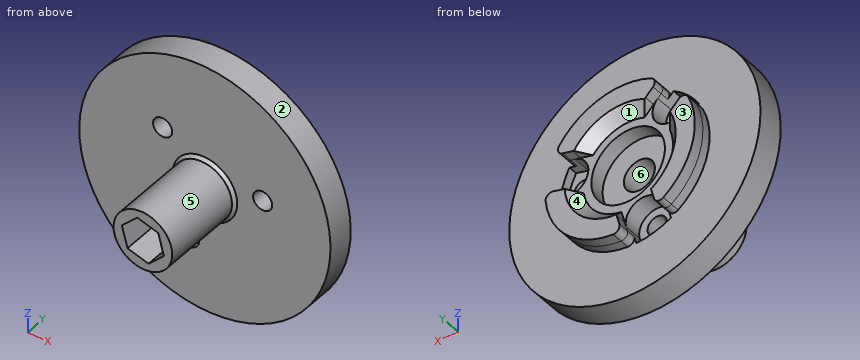
```python
from build123d import *
from build123d.topology import SkipClean

# Parameters (mm, degrees)
SKETCH_1_R               = 4
SKETCH_1_R_2             = 2.625
EXTRUDE_1_DEPTH          = 6
SKETCH_2_R               = 12.5
SKETCH_2_R_2             = 2.6
EXTRUDE_2_DEPTH          = 6
SKETCH_3_R               = 1.6
CUT_EXTRUDE_1_DEPTH      = 15
SKETCH_6_R               = 1.6
CUT_EXTRUDE_5_DEPTH      = 3
PATTERN_CIRCULAR_1_COUNT = 3
EXTRUDE_START            = 13.8
SKETCH_4_R               = 4.9
SKETCH_4_R_2             = 2.6
EXTRUDE_3_DEPTH          = 13.8
SKETCH_7_R               = 6.15
CUT_EXTRUDE_7_DEPTH      = 2.5
CUT_EXTRUDE_8_DEPTH      = 12.55
SKETCH_10_R              = 21
SKETCH_10_R_2            = 12.5
EXTRUDE_4_DEPTH          = 4.5
EXTRUDE_5_DEPTH          = 1.8
PATTERN_CIRCULAR_2_COUNT = 3
FILLET_1_R               = 1
CHAMFER_1_SIZE           = 0.5
CHAMFER_2_SIZE           = 2


with BuildPart() as part:
    # 草图1 → 凸台-拉伸1 (new body)
    with BuildSketch(Plane(origin=(0, 0, 0), x_dir=(1, 0, 0), z_dir=(0, 1, 0))):
        with Locations(Location((0, 0, 0), (0, 0, 270))):
            Circle(SKETCH_1_R)
        with Locations(Location((0, 0, 0), (0, 0, 270))):
            Circle(SKETCH_1_R_2, mode=Mode.SUBTRACT)
    extrude(amount=EXTRUDE_1_DEPTH)

    # 草图2 → 凸台-拉伸2 (add)
    with BuildSketch(Plane(origin=(0, 0, 0), x_dir=(-1, 0, 0), z_dir=(0, -1, 0))):
        with Locations(Location((0, 0, 0), (0, 0, 90))):
            Circle(SKETCH_2_R)
        with Locations(Location((0, 0, 0), (0, 0, 90))):
            Circle(SKETCH_2_R_2, mode=Mode.SUBTRACT)
    extrude(amount=-EXTRUDE_2_DEPTH)

    # 草图3 → 切除-拉伸1 (cut)
    with BuildSketch(Plane(origin=(0, 6, 0), x_dir=(1, 0, 0), z_dir=(0, 1, 0))):
        with Locations(Location((-2.588190451, 9.659258263, 0), (0, 0, 270))):
            Circle(SKETCH_3_R)
    cut_extrude_1 = extrude(amount=-CUT_EXTRUDE_1_DEPTH, mode=Mode.SUBTRACT)

    # 草图6 → 切除-拉伸5 (cut)
    with BuildSketch(Plane(origin=(0, 6, 0), x_dir=(1, 0, 0), z_dir=(0, 1, 0))):
        with BuildLine():
            Line((-6.038458877, 10.944725414), (-5.48596793, 8.882801128))
            ThreePointArc((-5.48596793, 8.882801128), (-1.811733316, 6.761480784), (0.309587028, 10.435715398))
            Line((0.309587028, 10.435715398), (-0.24290392, 12.497639685))
            ThreePointArc((-0.24290392, 12.497639685), (-3.235238064, 12.074072829), (-6.038458877, 10.944725414))
        make_face()
        with Locations(Location((-2.588190451, 9.659258263, 0), (0, 0, 270))):
            Circle(SKETCH_6_R, mode=Mode.SUBTRACT)
    cut_extrude_5 = extrude(amount=-CUT_EXTRUDE_5_DEPTH, mode=Mode.SUBTRACT)

    # 阵列(圆周)1: 切除-拉伸1, 切除-拉伸5 ×3 about axis
    pattern_circular_1_axis = Axis((0, 0, 0), (0, 1, 0))
    add([cut_extrude_1.rotate(pattern_circular_1_axis, i * 360 / PATTERN_CIRCULAR_1_COUNT) for i in range(1, PATTERN_CIRCULAR_1_COUNT)], mode=Mode.SUBTRACT)
    add([cut_extrude_5.rotate(pattern_circular_1_axis, i * 360 / PATTERN_CIRCULAR_1_COUNT) for i in range(1, PATTERN_CIRCULAR_1_COUNT)], mode=Mode.SUBTRACT)

    # 草图4 → 凸台-拉伸3 (add)
    with BuildSketch(Plane(origin=(0, 0, 0), x_dir=(-1, 0, 0), z_dir=(0, -1, 0)).offset(EXTRUDE_START)):
        with Locations(Location((0, 0, 0), (0, 0, 270))):
            Circle(SKETCH_4_R)
        with Locations(Location((0, 0, 0), (0, 0, 90))):
            Circle(SKETCH_4_R_2, mode=Mode.SUBTRACT)
    extrude(amount=-EXTRUDE_3_DEPTH)

    # 草图7 → 切除-拉伸7 (cut)
    with BuildSketch(Plane(origin=(0, 6, 0), x_dir=(1, 0, 0), z_dir=(0, 1, 0))):
        with Locations(Location((0, 0, 0), (0, 0, 270))):
            Circle(SKETCH_7_R)
    extrude(amount=-CUT_EXTRUDE_7_DEPTH, mode=Mode.SUBTRACT)

    # 草图8 → 切除-拉伸8 (cut)
    with BuildSketch(Plane(origin=(0, -13.8, 0), x_dir=(-1, 0, 0), z_dir=(0, -1, 0))):
        Polygon((-2.57196423, -2.57196423), (0.941404246, -3.513368476), (3.513368476, -0.941404246), (2.57196423, 2.57196423), (-0.941404246, 3.513368476), (-3.513368476, 0.941404246), align=None)
    extrude(amount=-CUT_EXTRUDE_8_DEPTH, mode=Mode.SUBTRACT)

    # 草图10 → 凸台-拉伸4 (add)
    with BuildSketch(Plane(origin=(0, 0, 0), x_dir=(1, 0, 0), z_dir=(0, 1, 0))):
        with Locations(Location((0, 0, 0), (0, 0, 270))):
            Circle(SKETCH_10_R)
        Circle(SKETCH_10_R_2, mode=Mode.SUBTRACT)
    extrude(amount=EXTRUDE_4_DEPTH)

    # 草图11 → 凸台-拉伸5 (add)
    with BuildSketch(Plane(origin=(0, 6, 0), x_dir=(1, 0, 0), z_dir=(0, 1, 0))):
        with BuildLine():
            Line((-5.230740824, 7.930280602), (-6.038458877, 10.944725414))
            ThreePointArc((-6.038458877, 10.944725414), (-12.074072829, 3.235238064), (-10.701821494, -6.459180807))
            Line((-10.701821494, -6.459180807), (-8.495094736, -4.252454048))
            ThreePointArc((-8.495094736, -4.252454048), (-9.17629535, 2.458780928), (-5.230740824, 7.930280602))
        make_face()
    extrude_5 = extrude(amount=EXTRUDE_5_DEPTH)

    # 阵列(圆周)2: 凸台-拉伸5 ×3 about axis
    with SkipClean():  # the faces are left unmerged after this step: merging them gives an invalid solid
        pattern_circular_2_axis = Axis((0, 3.5, 0), (0, 1, 0))
        for i in range(1, PATTERN_CIRCULAR_2_COUNT):
            add(extrude_5.rotate(pattern_circular_2_axis, i * 360 / PATTERN_CIRCULAR_2_COUNT))

    # 圆角1
    fillet_1_edges = [part.edges().sort_by_distance(p)[0] for p in [
        (-10.701821494, 6.9, 6.459180807),
        (-6.459180807, 6.9, 10.701821494),
        (10.944725414, 6.9, 6.038458877),
        (12.497639685, 6.9, 0.24290392),
        (-0.24290392, 6.9, -12.497639685),
        (-6.038458877, 6.9, -10.944725414),
    ]]
    fillet(fillet_1_edges, radius=FILLET_1_R)

    # 倒角1
    chamfer_1_edges = [part.edges().sort_by_distance(p)[0] for p in [
        (0, 0, -4.9),
    ]]
    chamfer(chamfer_1_edges, length=CHAMFER_1_SIZE)

    # 倒角2
    # the kernel refuses this chamfer: 2 mm, written as the material it adds along each edge
    with BuildSketch(Plane(origin=(0, 6, 0), x_dir=(-0.46364396793112084, 0, -0.8860215973671781), z_dir=(-0.8860215973671781, 0, 0.46364396793112084))) as chamfer_2_piece_1_section:
        Polygon((9.5 - CHAMFER_2_SIZE, 0), (9.5, -CHAMFER_2_SIZE), (9.5, 0), align=None)
    chamfer_2_piece_1 = revolve(axis=Axis((0, 6, 0), (0, -1, 0)), revolution_arc=145.244994466, mode=Mode.PRIVATE)
    chamfer_2_piece_1 = split(chamfer_2_piece_1, bisect_by=Plane(origin=(4.843261848, 6.879467901, -1.80808044), z_dir=(0.2588190451025276, 0, -0.9659258262890666)), keep=Keep.TOP, mode=Mode.PRIVATE)
    chamfer_2_piece_1 = split(chamfer_2_piece_1, bisect_by=Plane(origin=(1.80808044, 6.879467901, -4.843261848), z_dir=(0.9659258262890712, 0, -0.2588190451025102)), keep=Keep.TOP, mode=Mode.PRIVATE)
    chamfer_2_piece_1 = split(chamfer_2_piece_1, bisect_by=Plane(origin=(5.954215348, 7.8, -5.954215348), z_dir=(0, -1, 0)), keep=Keep.TOP, mode=Mode.PRIVATE)
    add(chamfer_2_piece_1)
    with BuildSketch(Plane(origin=(0, 6, 0), x_dir=(0.9991391955872041, 0, 0.04148334414382066), z_dir=(0.04148334414382066, 0, -0.9991391955872041))) as chamfer_2_piece_2_section:
        Polygon((9.5 - CHAMFER_2_SIZE, 0), (9.5, -CHAMFER_2_SIZE), (9.5, 0), align=None)
    chamfer_2_piece_2 = revolve(axis=Axis((0, 6, 0), (0, -1, 0)), revolution_arc=145.244994466, mode=Mode.PRIVATE)
    chamfer_2_piece_2 = split(chamfer_2_piece_2, bisect_by=Plane(origin=(3.290347577, 6.879467901, 3.987474517), z_dir=(-0.25881904510253106, 0, 0.9659258262890655)), keep=Keep.TOP, mode=Mode.PRIVATE)
    chamfer_2_piece_2 = split(chamfer_2_piece_2, bisect_by=Plane(origin=(-0.855787331, 6.879467901, 5.098428018), z_dir=(0.7071067811865428, 0, 0.7071067811865523)), keep=Keep.TOP, mode=Mode.PRIVATE)
    chamfer_2_piece_2 = split(chamfer_2_piece_2, bisect_by=Plane(origin=(2.179394077, 7.8, 8.133609425), z_dir=(0, -1, 0)), keep=Keep.TOP, mode=Mode.PRIVATE)
    add(chamfer_2_piece_2)
    with BuildSketch(Plane(origin=(0, 6, 0), x_dir=(-0.535495227656083, 0, 0.8445382532233574), z_dir=(0.8445382532233574, 0, 0.535495227656083))) as chamfer_2_piece_3_section:
        Polygon((9.5, -CHAMFER_2_SIZE), (9.5 - CHAMFER_2_SIZE, 0), (9.5, 0), align=None)
    chamfer_2_piece_3 = revolve(axis=Axis((0, 6, 0), (0, -1, 0)), revolution_arc=145.244994466, mode=Mode.PRIVATE)
    chamfer_2_piece_3 = split(chamfer_2_piece_3, bisect_by=Plane(origin=(-3.987474517, 6.879467901, -3.290347577), z_dir=(-0.96592582628907, 0, 0.25881904510251447)), keep=Keep.TOP, mode=Mode.PRIVATE)
    chamfer_2_piece_3 = split(chamfer_2_piece_3, bisect_by=Plane(origin=(-5.098428018, 6.879467901, 0.855787331), z_dir=(-0.7071067811865401, 0, -0.7071067811865549)), keep=Keep.TOP, mode=Mode.PRIVATE)
    chamfer_2_piece_3 = split(chamfer_2_piece_3, bisect_by=Plane(origin=(-8.133609425, 7.8, -2.179394077), z_dir=(0, -1, 0)), keep=Keep.TOP, mode=Mode.PRIVATE)
    add(chamfer_2_piece_3)


solid = part.part
```
CAD build for the part. Positions are in the model's coordinates, mm. Face numbers are marked on the shaded views. A direction names the side the tool comes from. Coordinates: 2 decimals unless noted, no trailing zeros. Order: outer loops, then holes, each group sorted by start corner. A loop starts at its lowest first (then second) coordinate and runs counter-clockwise, first axis right, second up. Notation, with made-up numbers: M -24.5,10.25 L 16.5,10.25 A24 cw 16.5,32.25 Z; hole C 35,-16 d8. An arc over 180 degrees is marked long. Write each question's results on one line, items separated by ' | '. Start each with the question number.
Q1. Flat gauge pins, fed straight in: P1, Ø6, axis at x = 0, z = 0, coming from the +Y side; P2, Ø3.5, axis at x = -7.07, z = 7.07, coming from the +Y side; P3, Ø1, axis at y = -9.5, z = 1, coming from the +X side; P4, Ø12.5, axis at x = -5, z = 5.5, coming from the -Y side. Where does each tip first touch, or does it go through?
Q2. Cut at B-B (x = -16). List the corners of the cut face in (y, z).
Q3. Cut at A-A (y = -4.5). List the corners of the cut face in (x, z).
Q4. Which spindle directions (+Z, -Z, +X, -X, +Y, -Y) get a long thin tool onto all of the face, cutting with end or side? Do the marked faces 4, 5 and 6. Say none if no direction does.
Q5. Pull direction X, two halves, no side cores. Call the marked faces 1, 2 and 3: +X half, -X half, draft (parallel to the pull), parting line (faces both ways), or undercut.
Q6. Drill centre lines: probe 1 along Z at (x, y) = (-1, 4); probe 2 along Z at (x, y) = (2.5, -3); probe 3 along Y at (x, z) = (-11, 2). Where is each one in solid material? Low to high. Write a range as from..to.
Found:
1) P1: y = 3.5 | P2: y = 3 | P3: x = 4.87 | P4: y = -13.8
2) outline: M 0,-13.6 L 4.5,-13.6 L 4.5,13.6 L 0,13.6 Z
3) outline: C 0,0 d9.8; hole M -3.51,0.94 L -2.57,-2.57 L 0.94,-3.51 L 3.51,-0.94 L 2.57,2.57 L -0.94,3.51 Z
4) face 4: +Y | face 5: -Y | face 6: +Y, -Y
5) face 1: undercut | face 2: parting line | face 3: draft
6) probe 1: -20.98..-12.46, -7.11..-6.07, 6.07..20.98 | probe 2: -4.21..-1.95, 2.59..4.21 | probe 3: 0..7.8
